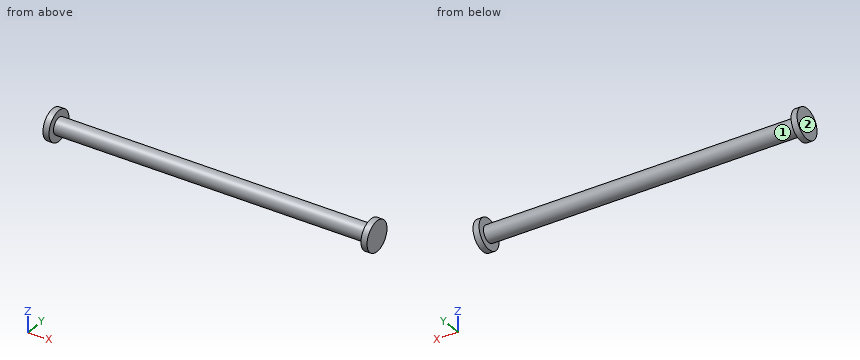
from build123d import *

# Parameters (mm, degrees)
F0_R     = 2.75
F1_DEPTH = 103.38
F2_R     = 5
F3_DEPTH = 2
F5_R     = 5
F6_DEPTH = 2


with BuildPart() as f1:
    # F0 (on Right) → F1 (new body)
    with BuildSketch(Plane.YZ):
        Circle(F0_R)
    extrude(amount=F1_DEPTH)

    # F2 (on Right) → F3 (join)
    with BuildSketch(Plane.YZ):
        Circle(F2_R)
    extrude(amount=-F3_DEPTH)

    # F5 (on offset) → F6 (join)
    with BuildSketch(Plane.YZ.offset(103.38)):
        Circle(F5_R)
    extrude(amount=F6_DEPTH)


solid = f1.part
Build history of the part. All positions in model axes, mm. Face numbers are marked on the shaded views. A direction names the side the tool comes from. Round coordinates to 2 decimals unless told otherwise and drop trailing zeros. Write each loop counter-clockwise with the first axis right and the second up, starting at its lowest first coordinate (ties: lowest second). Pieces come first, ordered by that corner, then holes. Notation, with made-up numbers: (48.5, 17) -> (59.5, 17) arc R29 ccw to (59.5, 47) -> close; hole circle Ø4 at (1.25, -31.75). An arc over 180 degrees is marked (long way). Use one line per item in the form item = value.
Q1. Band-saw the part on C-C, the plane x = 5.5. Write the cut outline in (y, z).
Conclusion:
outline = circle Ø5.5 at (0, 0)
Q2. Band-saw the part on A-A, the plane z = 0. Write the cut outline in (x, y).
Conclusion:
outline = (-2, -5) -> (0, -5) -> (0, -2.75) -> (103.38, -2.75) -> (103.38, -5) -> (105.38, -5) -> (105.38, 5) -> (103.38, 5) -> (103.38, 2.75) -> (0, 2.75) -> (0, 5) -> (-2, 5) -> close
Q3. Drill centre lines: L1, parallel to X at y = 4, z = 1; L2, parallel to Z at x = 13, y = -0.25; L3, parallel to Y at x = 38, z = -1.75. Where is each one in solid material? Low to high.
Conclusion:
L1 = -2 to 0, 103.38 to 105.38
L2 = -2.74 to 2.74
L3 = -2.12 to 2.12
Q4. Tool access for the marked faces 1 and 2: list every direction of +Z, -Z, +X, -X, +Y, -Y with a clear straight run to the whole face (end or side of a thin tool).
Conclusion:
face_1 = none
face_2 = +Z, -Z, -X, +Y, -Y
Q5. Drop flat-ended pins along their axis: P1, Ø5, axis at x = 62.5, z = -4, coming from the -Y side; P2, Ø1.5, axis at x = 22, z = -3, coming from the -Y side; P3, Ø1.5, axis at x = 78.5, y = 0, coming from the +Z side. Give the stop position or say it passes through.
Conclusion:
P1 = -2.3
P2 = -1.58
P3 = 2.75
